Source: CAD feature listing. Evaluate the final solid. Frame: model axes, mm. A direction names the side the tool comes from. Coordinates: 2 decimals unless noted, no trailing zeros. Order: outer loops, then holes, each group sorted by start corner. A loop starts at its lowest first (then second) coordinate and runs counter-clockwise, first axis right, second up. Notation, with made-up numbers: (58.5, -23.5) -> (102.5, -23.5) arc R8 cw to (102.5, -15.5) -> close; hole circle Ø7 at (52.25, -29.75). An arc over 180 degrees is marked (long way). Write item = value, one per line. Start each with the question number.
Item 1: Section query B-B (x = 0). Output: boundary loops of the cut face in (y, z).
Item 2: Section query D-D (z = 0). Output: boundary loops of the cut face in (x, y).
Item 3: Mould query, pull axis Z, two halves, no side actions, for faces 1 (the cylindrical face through (-0.4, -2.5, 43.5)), 2 (the flat face through (1, 0, -19)), 3 (the flat face through (-32.5, -0.8, -8)). Classes: released by +Z, released by -Z, zero draft, split by the parting line, or undercut.
Item 4: Ray query, line 1 along X through (y, z) = (-0.7, 0); line 2 along Y through (x, z) = (-8.5, 40); line 3 along X through (y, z) = (-0.7, -26.5). Return the intervals inside material, ascending. Write a range as [from, to].
Item 5: Contact query for flat-ended pins moving along their axis: pin 1 (4 mm diameter, centred on x = -4, z = -25, fed in from -Y); pin 2 (3 mm diameter, centred on y = -1, z = 23, fed in from +X); pin 3 (1.5 mm diameter, centred on x = -24.5, y = -3, fed in from +Z). Output: stop coordinate, or through.
Item 6: Section query C-C (z = 11.5). Output: boundary loops of the cut face in (x, y), then the cut area to 3 significant figures.
Item 7: Set-up query: faces 4 (the cylindrical face through (-37.78, -2.97, 17.17)), 5 (the flat face through (-33.444, -1.909, -25.666)), 6 (the flat face through (33.444, -1.909, 25.666)), 7 (the flat face through (-25.616, -1.909, -33.395)), 8 (the flat face through (25.616, -1.909, 33.395)). Return all of +Z, -Z, +X, -X, +Y, -Y with unobstructed straight access to the full face (end or side cutting, diameter ignored); none if empty.
```python
from build123d import *

# Parameters (mm, degrees)
F1_DEPTH = 1
F3_DEPTH = 5
F5_DEPTH = 5


with BuildPart() as f1:
    # F0 (on Front) → F1 (new body)
    with BuildSketch(Plane.XZ):
        with BuildLine():
            Line((-16.124515, -8), (-40.721616, -8))
            ThreePointArc((-40.721616, -8), (41.5, 0), (-40.721616, 8))
            Line((-40.721616, 8), (-16.124515, 8))
            ThreePointArc((-16.124515, 8), (18, 0), (-16.124515, -8))
        make_face()
    extrude(amount=F1_DEPTH)

    # F2 (on face) → F3 (join)
    with BuildSketch(Plane(origin=(0, 0, 0), x_dir=(-1, 0, 0), z_dir=(0, 1, 0))):
        with BuildLine():
            Line((40.721616, 8), (42.75804, 8))
            ThreePointArc((42.75804, 8), (-43.5, 0), (42.75804, -8))
            Line((42.75804, -8), (40.721616, -8))
            ThreePointArc((40.721616, -8), (-41.5, 0), (40.721616, 8))
        make_face()
    extrude(amount=-F3_DEPTH)

    # F4 (on face) → F5 (cut, through all)
    with BuildSketch(Plane(origin=(0, 0, 0), x_dir=(-1, 0, 0), z_dir=(0, 1, 0))):
        with BuildLine():
            Line((30.865846, -23.087671), (23.087671, -30.865846))
            Line((23.087671, -30.865846), (26.623205, -34.40138))
            ThreePointArc((26.623205, -34.40138), (30.759145, -30.759145), (34.40138, -26.623205))
            Line((34.40138, -26.623205), (30.865846, -23.087671))
        make_face()
        with BuildLine():
            Line((26.623205, 34.40138), (23.087671, 30.865846))
            Line((23.087671, 30.865846), (30.865846, 23.087671))
            Line((30.865846, 23.087671), (34.40138, 26.623205))
            ThreePointArc((34.40138, 26.623205), (30.759145, 30.759145), (26.623205, 34.40138))
        make_face()
        with BuildLine():
            Line((-34.40138, 26.623205), (-30.865846, 23.087671))
            Line((-30.865846, 23.087671), (-23.087671, 30.865846))
            Line((-23.087671, 30.865846), (-26.623205, 34.40138))
            ThreePointArc((-26.623205, 34.40138), (-30.759145, 30.759145), (-34.40138, 26.623205))
        make_face()
    extrude(amount=-F5_DEPTH, mode=Mode.SUBTRACT)


solid = f1.part
```
Computed:
q1.outline = (-5, -43.5) -> (0, -43.5) -> (0, -18) -> (-1, -18) -> (-1, -41.5) -> (-5, -41.5) -> close; (-5, 41.5) -> (-1, 41.5) -> (-1, 18) -> (0, 18) -> (0, 43.5) -> (-5, 43.5) -> close
q2.outline = (18, -1) -> (41.5, -1) -> (41.5, -5) -> (43.5, -5) -> (43.5, 0) -> (18, 0) -> close
q3.face_1 = released by +Z
q3.face_2 = zero draft
q3.face_3 = undercut
q4.line_1 = [18, 43.5]
q4.line_2 = [-1, 0]
q4.line_3 = [-34.5, -34.28], [-27.45, 34.5]
q5.pin_1 = -1
q5.pin_2 = 37.82
q5.pin_3 = 36.44
q6.outline = (-41.95, -5) -> (-39.87, -5) -> (-39.87, -1) -> (-13.85, -1) -> (-13.85, 0) -> (-41.95, 0) -> close; (13.85, -1) -> (39.87, -1) -> (39.87, -5) -> (41.95, -5) -> (41.95, 0) -> (13.85, 0) -> close
q6.area = 72.8 mm^2
q7.face_4 = -Y
q7.face_5 = -Z, +Y, -Y
q7.face_6 = +Z, +Y, -Y
q7.face_7 = -X, +Y, -Y
q7.face_8 = +X, +Y, -Y
